```python
from build123d import *

# Parameters (mm, degrees)
F1_DEPTH   = 45
F3_DEPTH   = 5
F5_DEPTH   = 2
F6_SIZE2   = 1.4106158457
F6_SIZE    = 8
F6_2_SIZE2 = 1.4106158457
F6_2_SIZE  = 8
F7_W       = 8
F7_H       = 8
F8_DEPTH   = 10
F9_R       = 1.6
F10_DEPTH  = 8


# Not quite as in the source:
# - a pattern or mirror of a feature is missing from the dataset's text; its kind, count and spacing are read off the source's solid


with BuildPart() as f1:
    # F0 (on Top) → F1 (new body)
    with BuildSketch(Plane.XY):
        Polygon((-5, -10), (-5, 0), (5, 0), (5, -10), (10, -10), (10, 0), (27.5, 0), (27.5, 5), (-27.5, 5), (-27.5, 0), (-10, 0), (-10, -10), align=None)
    extrude(amount=F1_DEPTH)

    # F2 (on face) → F3 (cut, through all)
    with BuildSketch(Plane.XZ):
        with BuildLine():
            Line((-16, 37), (-20, 37))
            ThreePointArc((-20, 37), (-22, 35), (-20, 33))
            Line((-20, 33), (-16, 33))
            ThreePointArc((-16, 33), (-14, 35), (-16, 37))
        make_face()
        with BuildLine():
            Line((-20, 8), (-16, 8))
            ThreePointArc((-16, 8), (-14, 10), (-16, 12))
            Line((-16, 12), (-20, 12))
            ThreePointArc((-20, 12), (-22, 10), (-20, 8))
        make_face()
    f3 = extrude(amount=-F3_DEPTH, mode=Mode.SUBTRACT)

    # F3_copies: F3 across plane
    add(f3.mirror(Plane(origin=(0, 0, 0), x_dir=(0, 0, 1), z_dir=(1, 0, 0))), mode=Mode.SUBTRACT)

    # F4 (on face) → F5 (cut)
    with BuildSketch(Plane.XZ):
        with BuildLine():
            Line((-16, 40.5), (-20, 40.5))
            ThreePointArc((-20, 40.5), (-25.5, 35), (-20, 29.5))
            Line((-20, 29.5), (-16, 29.5))
            ThreePointArc((-16, 29.5), (-10.5, 35), (-16, 40.5))
        make_face()
        with BuildLine():
            Line((-16, 15.5), (-20, 15.5))
            ThreePointArc((-20, 15.5), (-25.5, 10), (-20, 4.5))
            Line((-20, 4.5), (-16, 4.5))
            ThreePointArc((-16, 4.5), (-10.5, 10), (-16, 15.5))
        make_face()
    f5 = extrude(amount=-F5_DEPTH, mode=Mode.SUBTRACT)

    # F5_copies: F5 across plane
    add(f5.mirror(Plane(origin=(0, 0, 0), x_dir=(0, 0, 1), z_dir=(1, 0, 0))), mode=Mode.SUBTRACT)

    # F6
    f6_edges = [f1.edges().sort_by_distance(p)[0] for p in [
        (-5, -5, 45),
    ]]
    f6_side = f1.faces().sort_by_distance((-5, -5, 22.5))[0]
    chamfer(f6_edges, length=F6_SIZE, length2=F6_SIZE2, reference=f6_side)

    # F6#2
    f6_2_edges = [f1.edges().sort_by_distance(p)[0] for p in [
        (5, -5, 45),
    ]]
    f6_2_side = f1.faces().sort_by_distance((5, -5, 22.5))[0]
    chamfer(f6_2_edges, length=F6_2_SIZE, length2=F6_2_SIZE2, reference=f6_2_side)

    # F7 (on face) → F8 (join)
    with BuildSketch(Plane.XZ):
        with Locations((-23.5, 22.5)):
            Rectangle(F7_W, F7_H)
        with Locations((23.5, 22.5)):
            Rectangle(F7_W, F7_H)
    extrude(amount=F8_DEPTH)

    # F9 (on face) → F10 (cut, through all)
    with BuildSketch(Plane.XY.offset(26.5)):
        with Locations((-23.5, -6)):
            Circle(F9_R)
        with Locations((23.5, -6)):
            Circle(F9_R)
    extrude(amount=-F10_DEPTH, mode=Mode.SUBTRACT)


solid = f1.part
```
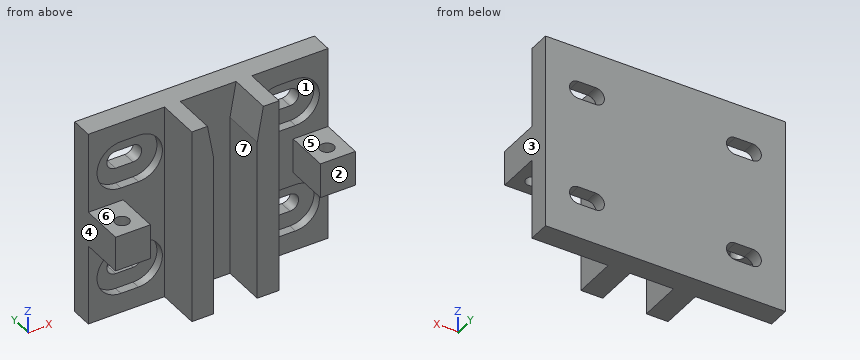
The model under review builds one solid part; all positions refer to its coordinate system, in mm. Face numbers are marked on the shaded views. A direction names the side the tool comes from. Give positions to 0.01 mm unless a question says otherwise; leave off trailing zeros. Write each loop counter-clockwise with the first axis right and the second up, starting at its lowest first coordinate (ties: lowest second). Pieces come first, ordered by that corner, then holes. Notation, with made-up numbers: (40.5, 29) -> (79.5, 29) arc R21 cw to (79.5, 46) -> close; hole circle Ø2 at (34.25, 4.5). An arc over 180 degrees is marked (long way). Answer in a Markdown table with one row per item.
1) Add section C-C on x = 17.5. State the section outline as (y, z) points.
Worked answers:
| item | result |
|---|---|
| outline | (0, 0) -> (5, 0) -> (5, 8) -> (2, 8) -> (2, 4.5) -> (0, 4.5) -> close; (0, 15.5) -> (2, 15.5) -> (2, 12) -> (5, 12) -> (5, 33) -> (2, 33) -> (2, 29.5) -> (0, 29.5) -> close; (0, 40.5) -> (2, 40.5) -> (2, 37) -> (5, 37) -> (5, 45) -> (0, 45) -> close |
2) Tool access review of the marked faces 5, 6 and 7: name each direction out of +Z, -Z, +X, -X, +Y, -Y from which nothing blocks a thin tool from reaching the whole face with its end or side.
Worked answers:
| item | result |
|---|---|
| face 5 | +Z, +X, -Y |
| face 6 | +Z, -X, -Y |
| face 7 | +Z, -Z, -Y |
3) Add section D-D on x = 23.5. State the section outline as (y, z) points, plus the area to 3 significant figures.
Worked answers:
| item | result |
|---|---|
| outline | (-10, 18.5) -> (-7.6, 18.5) -> (-7.6, 26.5) -> (-10, 26.5) -> close; (-4.4, 18.5) -> (0, 18.5) -> (0, 14.24) -> (2, 14.24) -> (2, 5.76) -> (0, 5.76) -> (0, 0) -> (5, 0) -> (5, 45) -> (0, 45) -> (0, 39.24) -> (2, 39.24) -> (2, 30.76) -> (0, 30.76) -> (0, 26.5) -> (-4.4, 26.5) -> close |
| area | 245 mm² |
4) Add section B-B on y = -6. State the section outline as (x, z) points.
Worked answers:
| item | result |
|---|---|
| outline | (-27.5, 18.5) -> (-25.1, 18.5) -> (-25.1, 26.5) -> (-27.5, 26.5) -> close; (-21.9, 18.5) -> (-19.5, 18.5) -> (-19.5, 26.5) -> (-21.9, 26.5) -> close; (-10, 0) -> (-5, 0) -> (-5, 37) -> (-6.41, 45) -> (-10, 45) -> close; (5, 0) -> (10, 0) -> (10, 45) -> (6.41, 45) -> (5, 37) -> close; (19.5, 18.5) -> (21.9, 18.5) -> (21.9, 26.5) -> (19.5, 26.5) -> close; (25.1, 18.5) -> (27.5, 18.5) -> (27.5, 26.5) -> (25.1, 26.5) -> close |
5) Add section A-A on z = 10. State the section outline as (x, y) points.
Worked answers:
| item | result |
|---|---|
| outline | (-27.5, 0) -> (-25.5, 0) -> (-25.5, 2) -> (-22, 2) -> (-22, 5) -> (-27.5, 5) -> close; (-14, 2) -> (-10.5, 2) -> (-10.5, 0) -> (-10, 0) -> (-10, -10) -> (-5, -10) -> (-5, 0) -> (5, 0) -> (5, -10) -> (10, -10) -> (10, 0) -> (10.5, 0) -> (10.5, 2) -> (14, 2) -> (14, 5) -> (-14, 5) -> close; (22, 2) -> (25.5, 2) -> (25.5, 0) -> (27.5, 0) -> (27.5, 5) -> (22, 5) -> close |
6) For L1, parallel to X at y = -4, z = 20; L2, parallel to X at y = -4.5, z = 13; L3, parallel to Y at x = -23.5, z = 20, list the stretches that pass through material, from the lowest coordinate up. Write a range as [from, to].
Worked answers:
| item | result |
|---|---|
| L1 | [-27.5, -19.5], [-10, -5], [5, 10], [19.5, 27.5] |
| L2 | [-10, -5], [5, 10] |
| L3 | [-10, -7.6], [-4.4, 5] |
7) Mouldability with a two-part tool opening along X and no side actions: class the marked faces 1, 2, 3 and 4 as +X half, -X half, draft (parallel to the pull), parting line (faces both ways), or undercut.
Worked answers:
| item | result |
|---|---|
| face 1 | undercut |
| face 2 | draft |
| face 3 | +X half |
| face 4 | -X half |
8) Clearance check with flat-ended pins moving along their axes: P1, Ø0.9, axis at x = -18.5, y = 3.5, coming from the -Z side; P2, Ø6, axis at y = -8.5, z = 37.5, coming from the -X side; P3, Ø4, axis at x = -23.5, y = -6, coming from the -Z side; P4, Ø4, axis at x = 23.5, y = -4.5, coming from the +Z side. State where each tip first meets the part, or that it passes through.
Worked answers:
| item | result |
|---|---|
| P1 | z = 0 |
| P2 | x = -10 |
| P3 | z = 18.5 |
| P4 | z = 26.5 |
